The listing builds one solid part. Answer for the finished solid, in the listing's coordinates (mm). Face numbers are marked on the shaded views. A direction names the side the tool comes from. Round coordinates to 2 decimals unless told otherwise and drop trailing zeros. Loops run counter-clockwise (first coordinate to the right, second up) from the corner with the lowest first, then second, coordinate; pieces in that order, holes last. Notation, with made-up numbers: M 4,-12.75 L 33,-12.75 A30 cw 33,21.25 Z; hole C 77.5,53.25 d10. An arc over 180 degrees is marked long. Answer as a JSON object with one key per item and string values.
```python
from build123d import *


with BuildPart() as part:
    # Sweep2: sweep along a path in Sketch12
    with BuildLine(Plane(origin=(0, 0, 0), x_dir=(1, 0, 0), z_dir=(0, 1, 0))) as sweep2_path:
        ThreePointArc((0, 0), (-0.074470784, -2.5), (-0.297619048, -4.99113443))
    # Sketch2 → Sweep2 (sweep)
    with BuildSketch(Plane.XY):
        with BuildLine():
            Line((-1.3, 7.7), (1.3, 7.7))
            Line((1.3, 7.7), (1.3, 5.2))
            ThreePointArc((1.3, 5.2), (1.229474497, 4.681174375), (1.023016035, 4.2))
            ThreePointArc((1.023016035, 4.2), (0.74603207, 3.2), (1.023016035, 2.2))
            ThreePointArc((1.023016035, 2.2), (1.229474497, 1.718825625), (1.3, 1.2))
            Line((1.3, 1.2), (1.3, -1.3))
            ThreePointArc((1.3, -1.3), (1.170809924, -1.635410197), (0.85, -1.797493719))
            ThreePointArc((0.85, -1.797493719), (0.529190076, -1.95957724), (0.4, -2.294987437))
            ThreePointArc((0.4, -2.294987437), (0.546446609, -2.648540828), (0.9, -2.794987437))
            Line((0.9, -2.794987437), (2.1, -2.794987437))
            ThreePointArc((2.1, -2.794987437), (2.453553391, -2.648540828), (2.6, -2.294987437))
            Line((2.6, -2.294987437), (2.6, 1.1))
            ThreePointArc((2.6, 1.1), (2.529474497, 1.618825625), (2.323016035, 2.1))
            ThreePointArc((2.323016035, 2.1), (1.982702832, 3.140572492), (2.258778081, 4.2))
            ThreePointArc((2.258778081, 4.2), (2.485981176, 4.628543914), (2.6, 5.1))
            Line((2.6, 5.1), (2.6, 8))
            ThreePointArc((2.6, 8), (2.307106781, 8.707106781), (1.6, 9))
            Line((1.6, 9), (-1.6, 9))
            ThreePointArc((-1.6, 9), (-2.307106781, 8.707106781), (-2.6, 8))
            Line((-2.6, 8), (-2.6, 5.1))
            ThreePointArc((-2.6, 5.1), (-2.485981176, 4.628543914), (-2.258778081, 4.2))
            ThreePointArc((-2.258778081, 4.2), (-1.982702832, 3.140572492), (-2.323016035, 2.1))
            ThreePointArc((-2.323016035, 2.1), (-2.529474497, 1.618825625), (-2.6, 1.1))
            Line((-2.6, 1.1), (-2.6, -2.294987437))
            ThreePointArc((-2.6, -2.294987437), (-2.453553391, -2.648540828), (-2.1, -2.794987437))
            Line((-2.1, -2.794987437), (-0.9, -2.794987437))
            ThreePointArc((-0.9, -2.794987437), (-0.546446609, -2.648540828), (-0.4, -2.294987437))
            ThreePointArc((-0.4, -2.294987437), (-0.529190076, -1.95957724), (-0.85, -1.797493719))
            ThreePointArc((-0.85, -1.797493719), (-1.170809924, -1.635410197), (-1.3, -1.3))
            Line((-1.3, -1.3), (-1.3, 1.2))
            ThreePointArc((-1.3, 1.2), (-1.229474497, 1.718825625), (-1.023016035, 2.2))
            ThreePointArc((-1.023016035, 2.2), (-0.74603207, 3.2), (-1.023016035, 4.2))
            ThreePointArc((-1.023016035, 4.2), (-1.229474497, 4.681174375), (-1.3, 5.2))
            Line((-1.3, 5.2), (-1.3, 7.7))
        make_face()
    sweep(path=sweep2_path.line)


solid = part.part
```
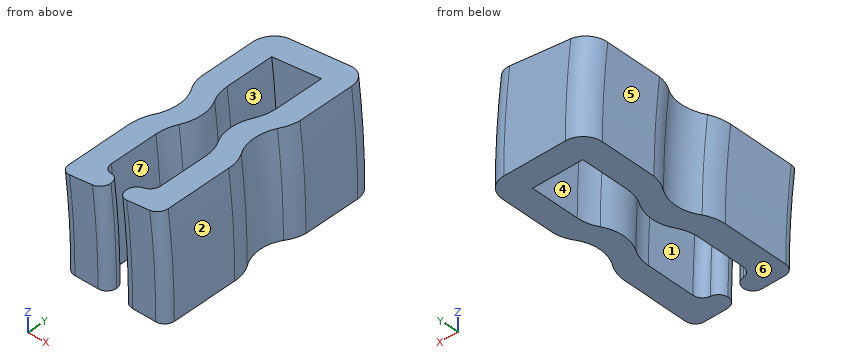
Item 1: Straight lines are drawn through the part: line 1 (Y direction, x = 0.95, z = 2.35); line 2 (X direction, y = 7.5, z = 4.15); line 3 (X direction, y = 7, z = 4.45). For each, find the intervals that lie inside material, in ascending order.
Values follow:
{"line 1": "-2.79 to -1.75, 2.21 to 4.19, 7.7 to 9", "line 2": "-2.82 to -1.51, 1.1 to 2.41", "line 3": "-2.85 to -1.54, 1.07 to 2.38"}
Item 2: A flat-ended cylindrical pin translates along its axis: P1, Ø1.5, axis at x = 1, y = -1, coming from the +Z side. Find the tip coordinate at first contact, or state that the pin passes through.
Values follow:
{"P1": "z = 5.24"}
Item 3: Determine the mould class of the marked faces 4, 5, 6 and 7 for opening direction X: released by +X, released by -X, zero draft, split by the parting line, or undercut.
Values follow:
{"face 4": "undercut", "face 5": "released by -X", "face 6": "zero draft", "face 7": "undercut"}
Item 4: Which of the six approach directions +Z, -Z, +X, -X, +Y, -Y give full straight-line access (tool end or side, diameter ignored) to the marked faces 1, 2 and 3?
Values follow:
{"face 1": "-Z", "face 2": "+Z, +X, +Y, -Y", "face 3": "+Z"}
Item 5: The part is cut by section A-A (y = 0.75). Give the vertices of the cut face in (x, z), then the cut area to 3 significant figures.
Values follow:
{"outline": "M -2.88,4.68 A39.4 cw -2.6,0 L -1.3,0 A40.7 ccw -1.59,4.84 Z; M 0.99,5.15 A43.3 cw 1.3,0 L 2.6,0 A44.6 ccw 2.28,5.3 Z", "area": "13.0 mm^2"}
Item 6: The part is cut by section B-B (y = 4.5). Give the vertices of the cut face in (x, z).
Values follow:
{"outline": "M -2.71,4.7 A39.57 cw -2.43,0 L -1.17,0 A40.83 ccw -1.46,4.85 Z; M 0.86,5.13 A43.17 cw 1.17,0 L 2.43,0 A44.43 ccw 2.12,5.28 Z"}
